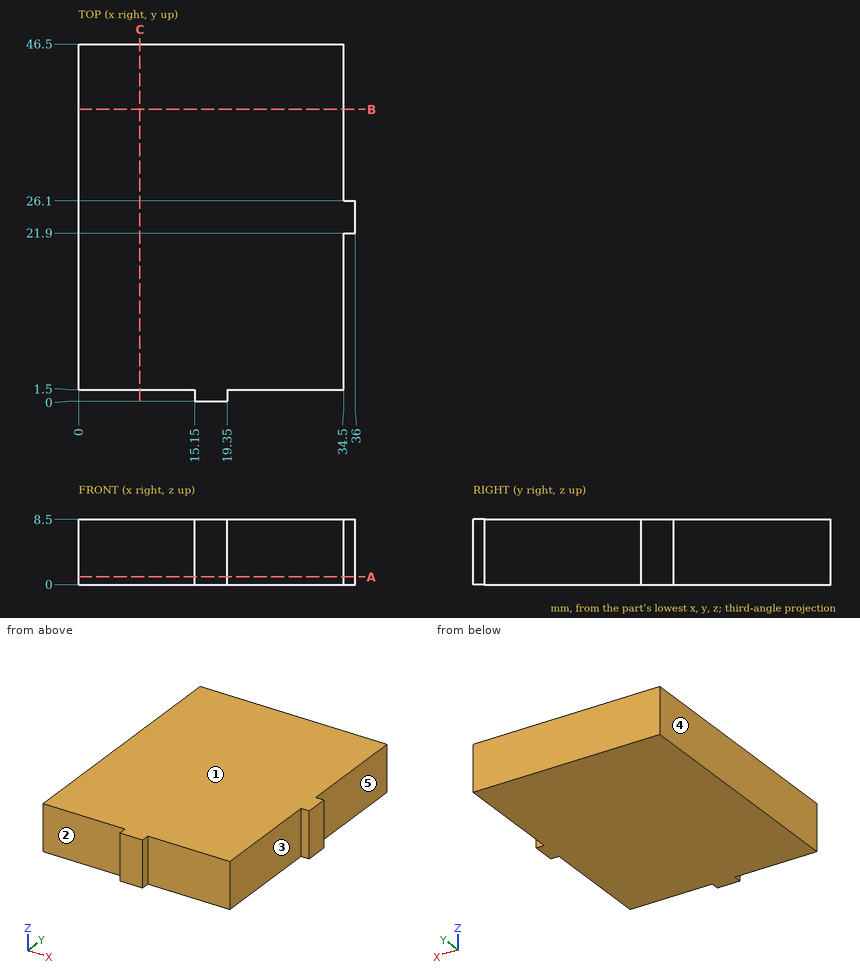
Study the drawing (mm; zero at the part's minimum x, y, z) and answer. A direction names the side the tool comes from. Coordinates: 2 decimals unless noted, no trailing zeros. Write each loop counter-clockwise with the first axis right and the second up, starting at its lowest first coordinate (ties: lowest second). Pieces come first, ordered by that corner, then holes. Notation, with made-up numbers: M 87.5,-26 L 145.5,-26 A14 ccw 145.5,-8 Z; hole C 58,79 d4. An arc over 180 degrees is marked long. Use one line per item in the form item = value.
Item 1: Find section B-B, the plane y = 38. Give the vertices of the cut face in (x, z), plus the area to 3 significant figures.
Model answer:
outline = M 0,0 L 34.5,0 L 34.5,8.5 L 0,8.5 Z
area = 293 mm2
Item 2: Find section A-A, the plane z = 1. Give the vertices of the cut face in (x, y).
Model answer:
outline = M 0,1.5 L 15.15,1.5 L 15.15,0 L 19.35,0 L 19.35,1.5 L 34.5,1.5 L 34.5,21.9 L 36,21.9 L 36,26.1 L 34.5,26.1 L 34.5,46.5 L 0,46.5 Z
Item 3: Find section C-C, the plane x = 8. Give the vertices of the cut face in (y, z), plus the area to 4 significant figures.
Model answer:
outline = M 1.5,0 L 46.5,0 L 46.5,8.5 L 1.5,8.5 Z
area = 382.5 mm2
Item 4: For the marked faces 1, 2, 3, 4 and 5, determine the directions among +Z, -Z, +X, -X, +Y, -Y from which every point of the face is accessible in a straight line to the end or side of a thin tool.
Model answer:
face_1 = +Z, +X, -X, +Y, -Y
face_2 = +Z, -Z, -X, -Y
face_3 = +Z, -Z, +X, -Y
face_4 = +Z, -Z, -X, +Y, -Y
face_5 = +Z, -Z, +X, +Y
Item 5: Given P1, Ø2.5, axis at y = 10.5, z = 4, coming from the +X side, flat-ended and moving along its own axis, determine where the tip first touches the part or whether it passes through.
Model answer:
P1 = 34.5
Item 6: Find the intervals of material crossed by probe 1 along Y at (x, z) = (2, 2); probe 2 along X at (y, z) = (6.5, 5), in increasing order.
Model answer:
probe_1 = 1.5 to 46.5
probe_2 = 0 to 34.5
